Verification items for the finished model (mm, model axes). Face numbers are marked on the shaded views. A direction names the side the tool comes from. Give positions to 0.01 mm unless a question says otherwise; leave off trailing zeros. Loops run counter-clockwise (first coordinate to the right, second up) from the corner with the lowest first, then second, coordinate; pieces in that order, holes last. Notation, with made-up numbers: (33.25, -2) - (46.25, -2) arc R28 cw to (46.25, 22) - close; hole circle Ø7 at (-34, 83). An arc over 180 degrees is marked (long way). One line per question, with ' | ' between items. Start each with the question number.
1. Thickness scan on line 1 along X through (y, z) = (15.5, 6.5); line 2 along X through (y, z) = (-5, -17.5); line 3 along X through (y, z) = (-4, 7.5). Record the ranges inside material, lowest first. Write a range as from..to.
2. Depth check by flat-ended pin: pin 1 Ø3 at (x, z) = (165.5, -14) entering from -Y; pin 2 Ø2 at (x, y) = (181.5, -4) entering from +Z; pin 3 Ø3 at (x, y) = (180.5, -15.5) entering from +Z. Enter the tip coordinate at first touch or a pass-through.
3. Section check A-A, the plane x = 181. Enter the section's corners in (y, z).
4. Tool access check on the marked faces 1 and 2. Record the directions out of +Z, -Z, +X, -X, +Y, -Y that give a thin tool (end or side, any length) a straight path to the whole face; none if there is none.
from build123d import *


with BuildPart() as part:
    # Sketch6 → Revolve1 (revolve)
    with BuildSketch(Plane.XY, mode=Mode.PRIVATE) as revolve1_sk:
        with BuildLine():
            Line((137, 2.5), (137, 0))
            Line((137, 0), (155, 0))
            Line((155, 0), (161.832507571, 0))
            Line((161.832507571, 0), (161.832507571, 13.982740363))
            Line((161.832507571, 13.982740363), (161.832507571, 21.4))
            Line((161.832507571, 21.4), (160.832507571, 21.4))
            Line((160.832507571, 21.4), (160.832507571, 20.4))
            Line((160.832507571, 20.4), (160.332507571, 20.4))
            Line((160.332507571, 20.4), (160.332507571, 21.4))
            Line((160.332507571, 21.4), (159.332507571, 21.4))
            ThreePointArc((159.332507571, 21.4), (158.150175861, 19.923922479), (156.5, 19))
            Line((156.5, 19), (156.5, 18))
            Line((156.5, 18), (155, 18))
            Line((155, 18), (155, 2.5))
            Line((155, 2.5), (137, 2.5))
        make_face()
        Polygon((161.832507571, 13.982740363), (161.832507571, 0), (162.539614352, 0), (162.539614352, 13.275633582), align=None)
        with BuildLine():
            Line((162.539614352, 13.275633582), (162.539614352, 0))
            Line((162.539614352, 0), (200, 0))
            Line((200, 0), (200, 2))
            Line((200, 2), (198, 2))
            Line((198, 2), (198, 19))
            Line((198, 19), (197.5, 19))
            ThreePointArc((197.5, 19), (196.497546245, 20.44777704), (195.016248395, 21.4))
            Line((195.016248395, 21.4), (194.539614352, 21.4))
            Line((194.539614352, 21.4), (194.539614352, 20.4))
            Line((194.539614352, 20.4), (194.039614352, 20.4))
            Line((194.039614352, 20.4), (194.039614352, 21.4))
            Line((194.039614352, 21.4), (193.039614352, 21.4))
            Line((193.039614352, 21.4), (193.039614352, 20.4))
            Line((193.039614352, 20.4), (192.539614352, 20.4))
            Line((192.539614352, 20.4), (192.539614352, 21.4))
            Line((192.539614352, 21.4), (162.539614352, 21.4))
            Line((162.539614352, 21.4), (162.539614352, 13.275633582))
        make_face()
    revolve(revolve1_sk.sketch.rotate(Axis((0, 0, 0), (1, 0, 0)), 90), axis=Axis((0, 0, 0), (1, 0, 0)))


solid = part.part
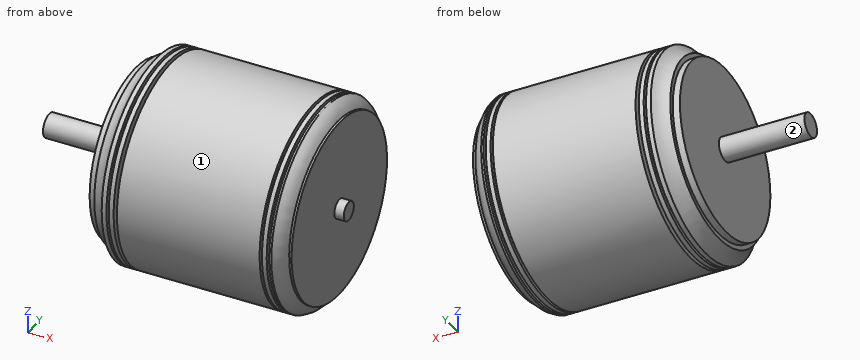
Results list:
1) line 1: 155..161.83, 162.54..198 | line 2: 156.5..161.83, 162.54..198 | line 3: 155..198
2) pin 1: y = -17.37 | pin 2: z = 21.19 | pin 3: z = 16.19
3) outline: circle Ø42.8 at (0, 0)
4) face 1: +X, -X | face 2: -X
